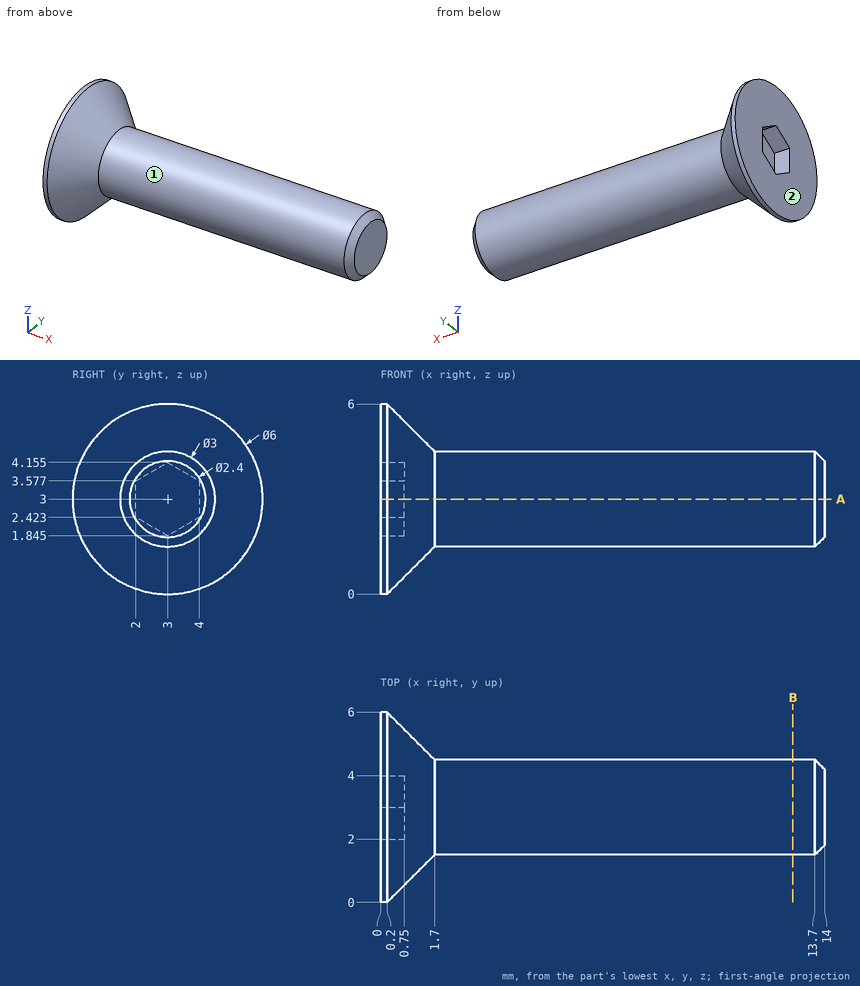
Answer from the drawing. Dimensions are ordinates in mm from the lowest x, y and z of the part. A direction names the side the tool comes from. Round coordinates to 2 decimals unless told otherwise and drop trailing zeros. Order: outer loops, then holes, each group sorted by start corner. A loop starts at its lowest first (then second) coordinate and runs counter-clockwise, first axis right, second up.
1) Flat-ended cylindrical pins translate along their axes: pin 1 (3 mm diameter, centred on x = 8, y = 1, fed in from -Z); pin 2 (2 mm diameter, centred on x = 2, z = 5, fed in from -Y); pin 3 (1 mm diameter, centred on x = 7, y = 2.5, fed in from +Z). Find the tip coordinate at first contact, or state that the pin passes through.
2) The part is cut by section A-A on z = 3. Write down the section's boundary in (x, y).
3) For the marked faces 1 and 2, determine the directions among +Z, -Z, +X, -X, +Y, -Y from which every point of the face is accessible in a straight line to the end or side of a thin tool.
4) The part is cut by section B-B on x = 13. Write down the section's boundary in (y, z).
5) Straight lines are drawn through the part: L1, parallel to Y at x = 5.5, z = 2.95; L2, parallel to Z at x = 0.75, y = 4.75 (1 decimal); L3, parallel to X at y = 1.55, z = 4.5 (1 decimal). For each, find the intervals that lie inside material, in ascending order.
Resolved:
1. pin 1: stops at z = 1.59
1. pin 2: stops at y = 1.57
1. pin 3: stops at z = 4.5
2. outline: (0, 0) - (0.2, 0) - (1.7, 1.5) - (13.7, 1.5) - (14, 1.8) - (14, 4.2) - (13.7, 4.5) - (1.7, 4.5) - (0.2, 6) - (0, 6) - (0, 4) - (0.75, 4) - (0.75, 2) - (0, 2) - close
3. face 1: +X
3. face 2: +Z, -Z, -X, +Y, -Y
4. outline: circle Ø3 at (3, 3)
5. L1: y = 1.5 to 4.5
5. L2: z = 1.3 to 4.7
5. L3: x = 0 to 1.1
